Design review of the part shown in the three views and the two pictorial views. Dimensions are in mm from the part's minimum x, y and z. A direction names the side the tool comes from. Round coordinates to 2 decimals unless told otherwise and drop trailing zeros. Write each loop counter-clockwise with the first axis right and the second up, starting at its lowest first coordinate (ties: lowest second). Pieces come first, ordered by that corner, then holes. Notation, with made-up numbers: (-7, 38) - (39, 38) arc R30 cw to (39, 71) - close; hole circle Ø11 at (65, 40). An arc over 180 degrees is marked (long way). Use one line per item in the form item = value.
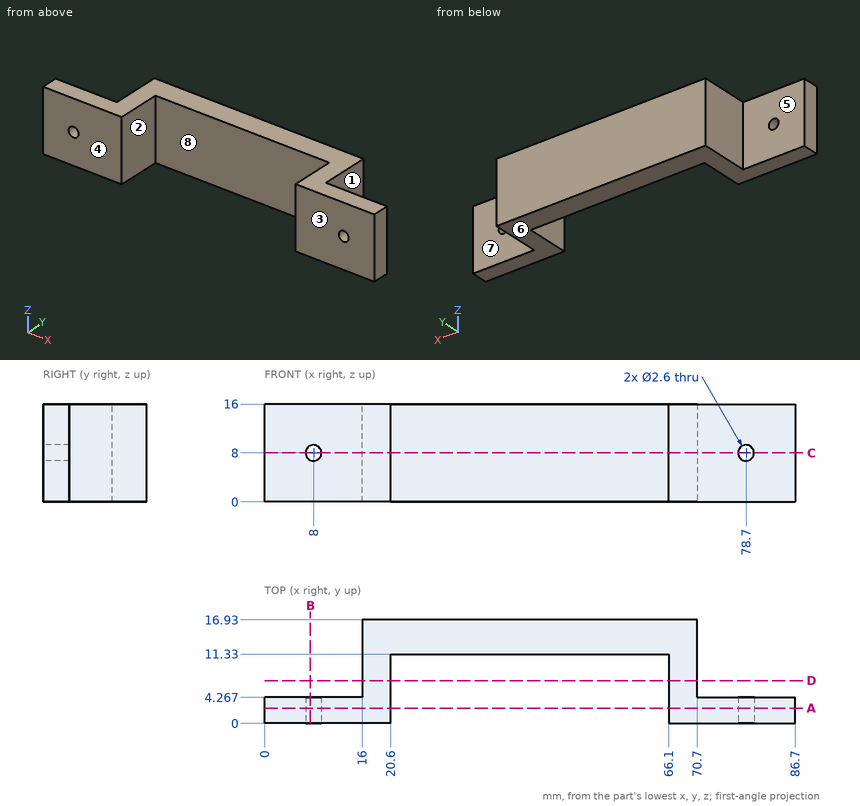
(1) Add section A-A on y = 2.5. Write out the cut boundary in (x, z).
Geometry results:
outline = (0, 0) - (20.6, 0) - (20.6, 16) - (0, 16) - close; (66.1, 0) - (86.7, 0) - (86.7, 16) - (66.1, 16) - close; hole circle Ø2.6 at (8, 8); hole circle Ø2.6 at (78.7, 8)
(2) Machinability: for the marked faces 4, 5, 6, 7 and 8, which of the approach directions +Z, -Z, +X, -X, +Y, -Y give a long, thin tool a straight path to every point of the face, cutting with its end or side? Answer none if there is none.
Geometry results:
face_4 = +Z, -Z, +X, -X, -Y
face_5 = +Z, -Z, -X, +Y
face_6 = -Z, +X, -X, +Y, -Y
face_7 = +Z, -Z, +X, +Y
face_8 = +Z, -Z, -Y
(3) Add section C-C on z = 8. Write out the cut boundary in (x, y).
Geometry results:
outline = (0, 0) - (6.7, 0) - (6.7, 4.27) - (0, 4.27) - close; (9.3, 0) - (20.6, 0) - (20.6, 11.33) - (66.1, 11.33) - (66.1, 0) - (77.4, 0) - (77.4, 4.27) - (70.7, 4.27) - (70.7, 16.93) - (16, 16.93) - (16, 4.27) - (9.3, 4.27) - close; (80, 0) - (86.7, 0) - (86.7, 4.27) - (80, 4.27) - close
(4) The part is to be moulded in two halves that separate along X. For the marked faces 1, 2 and 3, say which applies: +X half, -X half, draft (parallel to the pull), parting line (faces both ways), or undercut.
Geometry results:
face_1 = +X half
face_2 = undercut
face_3 = draft
(5) Add section D-D on y = 7. Write out the cut boundary in (x, z).
Geometry results:
outline = (16, 0) - (20.6, 0) - (20.6, 16) - (16, 16) - close; (66.1, 0) - (70.7, 0) - (70.7, 16) - (66.1, 16) - close
(6) Insertion check: P1, Ø5, axis at x = 12.5, z = 10.5, coming from the +Y side; P2, Ø2.5, axis at x = 8, z = 8, coming from the -Y side; P3, Ø2, axis at y = 8, z = 5.5, coming from the -X side. Each pin has a flat end and moves straight along its axis. Give the tip position at first contact, or say it passes through.
Geometry results:
P1 = 4.27
P2 = through
P3 = 16
(7) To check wall thickness, follow L1, parallel to X at y = 1.9, z = 8; L2, parallel to X at y = 9, z = 14.25; L3, parallel to Z at x = 8, y = 2.15. State the ranges of each line that lie inside material, in increasing order.
Geometry results:
L1 = 0 to 6.7, 9.3 to 20.6, 66.1 to 77.4, 80 to 86.7
L2 = 16 to 20.6, 66.1 to 70.7
L3 = 0 to 6.7, 9.3 to 16
(8) Add section B-B on x = 7.5. Write out the cut boundary in (y, z).
Geometry results:
outline = (0, 0) - (4.27, 0) - (4.27, 6.8) - (0, 6.8) - close; (0, 9.2) - (4.27, 9.2) - (4.27, 16) - (0, 16) - close
